Source: CAD feature listing. Evaluate the final solid. Frame: model axes, mm. Face numbers are marked on the shaded views. A direction names the side the tool comes from. Coordinates: 2 decimals unless noted, no trailing zeros. Order: outer loops, then holes, each group sorted by start corner. A loop starts at its lowest first (then second) coordinate and runs counter-clockwise, first axis right, second up.
Item 1: Reachability of the marked faces 1, 2 and 3 from +Z, -Z, +X, -X, +Y, -Y: full face, straight path, thin tool, end or side. Return the list, or none.
Item 2: Section B-B on z = 0. Return the cut outline in (x, y) (3 decimals).
Item 3: Section D-D on z = -5.75. Return the cut outline in (x, y) (3 decimals).
Item 4: Contact query for flat-ended pins moving along their axis: P1, Ø2.5, axis at x = 0, z = 6.1, coming from the -Y side; P2, Ø2, axis at x = -2, y = 8.5, coming from the -Z side; P3, Ø1.8, axis at y = 1, z = 0, coming from the -X side (3 decimals); P4, Ø1.8, axis at y = 0.5, z = -1, coming from the +X side (3 decimals). Output: stop coordinate, or through.
Item 5: Section A-A on x = 0. State how many separate pieces and enclosed holes the cut face has, then the cut area to 3 significant figures.
Item 6: Section C-C on y = 7. Return the cut outline in (x, z) (3 decimals).
Item 7: Mould query, pull axis Y, two halves, no side actions, for the marked faces 4, 5 and 6. Classes: released by +Y, released by -Y, zero draft, split by the parting line, or undercut.
Item 8: Ray query, line 1 (Z direction, x = 0, y = 5.25) (3 decimals); line 2 (Z direction, x = 0, y = 3.25); line 3 (Y direction, x = 0.5, z = 4.5). Return the intervals inside material, ascending.
Autodesk Inventor part; units mm, degrees
ref_plane "YZ Plane" through (0, 0, 0) normal (1, 0, 0) x (0, 1, 0)
ref_plane "XZ Plane" through (0, 0, 0) normal (0, 1, 0) x (-1, 0, 0)
ref_plane "XY Plane" through (0, 0, 0) normal (0, 0, 1) x (1, 0, 0)
sketch "Sketch10" plane through (0, 0, 0) normal (0, 0, 1) x (1, 0, 0)
  line L0 (-2, 0) -> (-8, 0)
  line L1 (-8, 0) -> (-8, 1.6)
  line L2 (-8, 1.6) -> (-2.65, 1.6)
  line L3 (-2.65, 1.6) -> (-2.65, 4.7)
  line L4 (-2.65, 4.7) -> (-3.175, 4.7)
  line L5 (-3.175, 4.7) -> (-3.175, 8.7)
  line L6 (-2, 7.6) -> (-2, 0)
  line L7 (-3.175, 8.7) -> (-2.65, 8.7)
  line L8 (-2.65, 8.7) -> (-2.65, 9.5)
  line L9 (-2.65, 9.5) -> (-2.325, 9.5)
  line L10 (0, -1.9) -> (0, 11.4)
  line L11 (-2.325, 9.5) -> (-2.325, 7.6)
  line L12 (-2.325, 7.6) -> (-2, 7.6)
  point P0 (0, 0)
  dimension "d39" = 2
  dimension "d41" = 0.8
  dimension "d42" = 4
  dimension "d43" = 2.65
  dimension "d44" = 1.6
  dimension "d45" = 8
  dimension "d46" = 3.175
  dimension "d66" = 2.325
  dimension "d67" = 1.9
  dimension "d68" = 9.5
revolve "Revolution1" add sketch "Sketch10" angle 360 about axis through (0, -10, 0) along (0, 1, 0)
sketch "Sketch11" plane through (0, 0, 0) normal (0, -1, 0) x (1, 0, 0)
  circle A0 centre (0, 0) radius 8
  line L0 (2.825, -7.4846) -> (2.825, 7.4846)
  line L1 (-2.825, -7.4846) -> (-2.825, 7.4846)
  arc A1 (2.825, -7.4846) -> (2.825, 7.4846) centre (0, 0) ccw
  arc A2 (-2.825, 7.4846) -> (-2.825, -7.4846) centre (0, 0) ccw
  dimension "d48" = 5.65
extrude "Extrusion7" cut sketch "Sketch11" against normal up to surface (1.6 mm away) contours A0 L0 | L1 A0
sketch "Sketch12" plane through (0, 0, 0) normal (0, -1, 0) x (1, 0, 0)
  line L0 (2.825, 7.4846) -> (2.825, -7.4846)
  line L1 (2.825, 6) -> (0.8727, 7.9523)
  line L2 (2.825, -6) -> (0.8727, -7.9523)
  arc A0 (-2.825, -7.4846) -> (2.825, -7.4846) centre (0, 0) ccw
  arc A1 (2.825, 7.4846) -> (-2.825, 7.4846) centre (0, 0) ccw
  line L3 (0, -11.2) -> (0, 11.2)
  line L4 (-2.825, 6) -> (-0.8727, 7.9523)
  line L5 (-2.825, -6) -> (-0.8727, -7.9523)
  line L6 (-2.825, 7.4846) -> (-2.825, -7.4846)
  dimension "d51" = 12
  dimension "d52" = 6
  dimension "d53" = 45
  dimension "d54" = 45
extrude "Extrusion8" cut sketch "Sketch12" against normal through all contours L0 L1 A1 | L0 A0 L2 | L4 L6 A1 | A0 L6 L5
sketch "Sketch13" plane through (0, 0, 0) normal (0, -1, 0) x (1, 0, 0)
  point P0 (0, 0)
  point P1 (0, 6.1)
  point P2 (0, -6.1)
  dimension "d57" = 12.2
  dimension "d58" = 6.1
hole "Hole3" at (0, 0, 6.1) at (0, 0, -6.1) direction (0, 1, 0) diameter 2.6 end through all
thread "Thread2"
equation "\"d54\" = d53"
properties part number "SMA-PanelMount-Ni-AuPlated-Body" material "Brass"
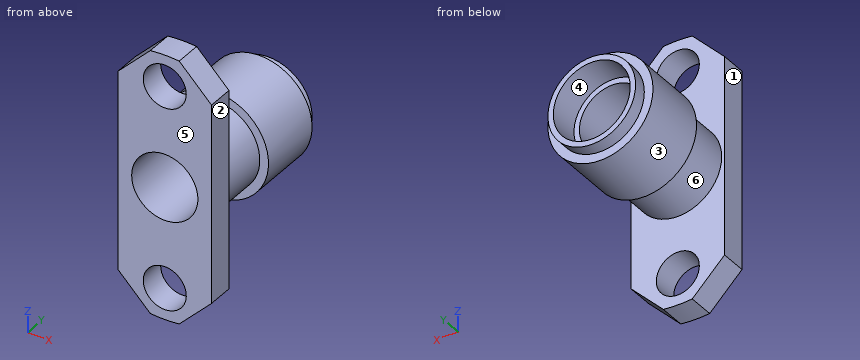
Answer list:
1. face 1: +Z, -Z, -X, -Y
1. face 2: +Z, -Z, +X, -Y
1. face 3: +Y
2. outline: (-3.175, 4.7) - (-2.65, 4.7) - (-2.65, 1.6) - (-2.825, 1.6) - (-2.825, 0) - (-2, 0) - (-2, 7.6) - (-2.325, 7.6) - (-2.325, 9.5) - (-2.65, 9.5) - (-2.65, 8.7) - (-3.175, 8.7) - close; (2, 0) - (2.825, 0) - (2.825, 1.6) - (2.65, 1.6) - (2.65, 4.7) - (3.175, 4.7) - (3.175, 8.7) - (2.65, 8.7) - (2.65, 9.5) - (2.325, 9.5) - (2.325, 7.6) - (2, 7.6) - close
3. outline: (-2.825, 0) - (-1.252, 0) - (-1.252, 1.6) - (-2.825, 1.6) - close; (1.252, 0) - (2.825, 0) - (2.825, 1.6) - (1.252, 1.6) - close
4. P1: passes through
4. P2: stops at z = -3.01
4. P3: stops at x = -2.825
4. P4: stops at x = 2.825
5. separate pieces: 4
5. enclosed holes: 0
5. area: 24.1 mm2
6. outline: circle Ø6.35 at (0, 0); hole circle Ø4 at (0, 0)
7. face 4: zero draft
7. face 5: released by -Y
7. face 6: undercut
8. line 1: z = -3.175 to -2, 2 to 3.175
8. line 2: z = -2.65 to -2, 2 to 2.65
8. line 3: y = 0 to 1.6
